from build123d import *

# Parameters (mm, degrees)
SKETCH1_W               = 50
SKETCH1_H               = 70
BOSS_EXTRUDE1_DEPTH     = 3
SKETCH2_R               = 6.5
CUT_EXTRUDE1_DEPTH      = 1
CUT_EXTRUDE1_DEPTH_BACK = 4
CUT_EXTRUDE2_DEPTH      = 1
CUT_EXTRUDE2_DEPTH_BACK = 4
SKETCH4_W               = 13
SKETCH4_H               = 15
CUT_EXTRUDE3_DEPTH      = 1
CUT_EXTRUDE3_DEPTH_BACK = 4
FILLET1_R               = 20


with BuildPart() as part:
    # Sketch1 → Boss-Extrude1 (new body)
    with BuildSketch(Plane.XY):
        with Locations((0, 5)):
            Rectangle(SKETCH1_W, SKETCH1_H)
    extrude(amount=BOSS_EXTRUDE1_DEPTH)

    # Sketch2 → Cut-Extrude1 (cut, two sides)
    with BuildSketch(Plane.XY.offset(3)) as cut_extrude1_sk:
        Circle(SKETCH2_R)
    extrude(amount=CUT_EXTRUDE1_DEPTH, mode=Mode.SUBTRACT)
    extrude(cut_extrude1_sk.sketch, amount=-CUT_EXTRUDE1_DEPTH_BACK, mode=Mode.SUBTRACT)

    # Sketch3 → Cut-Extrude2 (cut, two sides)
    with BuildSketch(Plane.XY.offset(3)) as cut_extrude2_sk:
        with BuildLine():
            Line((-5, 35), (5, 35))
            ThreePointArc((5, 35), (20, 20), (5, 5))
            Line((5, 5), (-5, 5))
            ThreePointArc((-5, 5), (-20, 20), (-5, 35))
        make_face()
    extrude(amount=CUT_EXTRUDE2_DEPTH, mode=Mode.SUBTRACT)
    extrude(cut_extrude2_sk.sketch, amount=-CUT_EXTRUDE2_DEPTH_BACK, mode=Mode.SUBTRACT)

    # Sketch4 → Cut-Extrude3 (cut, two sides)
    with BuildSketch(Plane.XY.offset(3)) as cut_extrude3_sk:
        with Locations((0, 7.5)):
            Rectangle(SKETCH4_W, SKETCH4_H)
    extrude(amount=CUT_EXTRUDE3_DEPTH, mode=Mode.SUBTRACT)
    extrude(cut_extrude3_sk.sketch, amount=-CUT_EXTRUDE3_DEPTH_BACK, mode=Mode.SUBTRACT)

    # Fillet1
    fillet1_edges = [part.edges().sort_by_distance(p)[0] for p in [
        (-25, 40, 1.5),
        (25, 40, 1.5),
    ]]
    fillet(fillet1_edges, radius=FILLET1_R)


solid = part.part
Source: CAD feature listing. Evaluate the final solid. Frame: model axes, mm. A direction names the side the tool comes from. Coordinates: 2 decimals unless noted, no trailing zeros. Order: outer loops, then holes, each group sorted by start corner. A loop starts at its lowest first (then second) coordinate and runs counter-clockwise, first axis right, second up.
Item 1: First-contact query: P1, Ø5, axis at x = -14.5, y = -0.5, coming from the -Z side; P2, Ø1.5, axis at x = -19.5, z = 1.5, coming from the +Y side. Flat tips, straight axial feed; report the tip coordinate or a pass-through.
Output values:
P1: stops at z = 0
P2: stops at y = 34.52
Item 2: Cut plane B-B (y = 8). Return loops of the section in (x, z).
Output values:
outline: (-25, 0) - (-14, 0) - (-14, 3) - (-25, 3) - close; (14, 0) - (25, 0) - (25, 3) - (14, 3) - close
Item 3: Set-up query: faces 1 (the face through (0, -10, 0)), 2 (the face through (6.5, 3, 2)). Return all of +Z, -Z, +X, -X, +Y, -Y with unobstructed straight access to the full face (end or side cutting, diameter ignored); none if empty.
Output values:
face 1: -Z, +X, -X, +Y, -Y
face 2: +Z, -Z
Item 4: Cut plane C-C (x = -17.5). Return loops of the section in (y, z).
Output values:
outline: (-30, 0) - (11.71, 0) - (11.71, 3) - (-30, 3) - close; (28.29, 0) - (35.61, 0) - (35.61, 3) - (28.29, 3) - close
Item 5: Pull-direction query (X, two-part tool) for faces 3 (the face through (0, -30, 1)), 4 (the face through (-6.5, 3, 2)), 5 (the face through (-19.297, 33.986, 1.521)); classes: pulls with the +X half, pulls with the -X half, needs draft (parallel to the pull), parting line crosses it, or undercut.
Output values:
face 3: needs draft
face 4: undercut
face 5: pulls with the -X half
Item 6: Material intervals for line 1 (X direction, y = 4.5, z = 1.35); line 2 (Y direction, x = 2, z = 1.85); line 3 (X direction, y = 27, z = 0.75) (1 decimal), sorted ascending.
Output values:
line 1: x = -25 to -6.5, 6.5 to 25
line 2: y = -30 to -6.18, 35 to 40
line 3: x = -23.7 to -18.3, 18.3 to 23.7
Item 7: Cut plane A-A (z = 1). Return loops of the section in (x, y), plus the area to 3 significant figures.
Output values:
outline: (-25, -30) - (25, -30) - (25, 20) arc R20 ccw to (5, 40) - (-5, 40) arc R20 ccw to (-25, 20) - close; hole (-6.5, 0) arc R6.5 ccw to (6.5, 0) - (6.5, 5.08) arc R15 ccw to (5, 35) - (-5, 35) arc R15 ccw to (-6.5, 5.08) - close
area: 2,190 mm2
